```python
from build123d import *

# Parameters (mm, degrees)
SKETCH1_R           = 114.3
SKETCH1_R_2         = 22.5
SKETCH1_R_3         = 30
BOSS_EXTRUDE1_DEPTH = 50
CUT_EXTRUDE1_START  = -35
SKETCH2_R           = 90
SKETCH2_R_2         = 60
CUT_EXTRUDE1_DEPTH  = 20


with BuildPart() as part:
    # Sketch1 → Boss-Extrude1 (new body)
    with BuildSketch(Plane(origin=(0, 0, 0), x_dir=(1, 0, 0), z_dir=(0, 1, 0))):
        with Locations(Location((0, 0, 0), (0, 0, 270))):
            Circle(SKETCH1_R)
        with Locations(Location((75, 0, 0), (0, 0, 270))):
            Circle(SKETCH1_R_2, mode=Mode.SUBTRACT)
        with Locations(Location((53.031031744, 53.03498536, 0), (0, 0, 270))):
            Circle(SKETCH1_R_2, mode=Mode.SUBTRACT)
        with Locations(Location((0, 75, 0), (0, 0, 270))):
            Circle(SKETCH1_R_2, mode=Mode.SUBTRACT)
        with Locations(Location((-52.573136336, 53.488927226, 0), (0, 0, 270))):
            Circle(SKETCH1_R_2, mode=Mode.SUBTRACT)
        with Locations(Location((-75, 0, 0), (0, 0, 270))):
            Circle(SKETCH1_R_2, mode=Mode.SUBTRACT)
        with Locations(Location((-53.03498536, -53.031031744, 0), (0, 0, 270))):
            Circle(SKETCH1_R_2, mode=Mode.SUBTRACT)
        with Locations(Location((0, -75, 0), (0, 0, 270))):
            Circle(SKETCH1_R_2, mode=Mode.SUBTRACT)
        with Locations(Location((53.488927226, -52.573136336, 0), (0, 0, 270))):
            Circle(SKETCH1_R_2, mode=Mode.SUBTRACT)
        with Locations(Location((0, 0, 0), (0, 0, 270))):
            Circle(SKETCH1_R_3, mode=Mode.SUBTRACT)
    extrude(amount=BOSS_EXTRUDE1_DEPTH)

    # Sketch2 → Cut-Extrude1 (cut)
    with BuildSketch(Plane(origin=(0, 50, 0), x_dir=(1, 0, 0), z_dir=(0, 1, 0)).offset(CUT_EXTRUDE1_START)):
        Circle(SKETCH2_R)
        Circle(SKETCH2_R_2, mode=Mode.SUBTRACT)
    extrude(amount=-CUT_EXTRUDE1_DEPTH, mode=Mode.SUBTRACT)


solid = part.part
```
The listing builds one solid part. Answer for the finished solid, in the listing's coordinates (mm). A direction names the side the tool comes from. Coordinates: 2 decimals unless noted, no trailing zeros. Loops run counter-clockwise (first coordinate to the right, second up) from the corner with the lowest first, then second, coordinate; pieces in that order, holes last. Notation, with made-up numbers: M 89.5,0.5 L 96.5,0.5 A23 cw 96.5,29.5 Z; hole C -39,27.25 d4. An arc over 180 degrees is marked long. Answer as CSV lines item,"result". Start each with the question number.
(1) The part is cut by section A-A (x = 0). Give the vertices of the cut face in (y, z).
(2) The part is cut by section D-D (z = -92). Give the vertices of the cut face in (x, y), and give its area (3 significant figures).
(3) The part is cut by section B-B (y = 5.5). State how many separate pieces and enclosed holes the cut face has, and give its area (3 significant figures).
(4) The mould has two halves that part along Z. Classify faces 3 (the flat face through (70, 15, -29)), 4 (the cylindrical face through (5.03, 24.65, -114.19)), 5 (the flat face through (27, 0, -27)): pulls with the +Z half, pulls with the -Z half, needs draft (parallel to the pull), parting line crosses it, or undercut.
(5) Given pin 1 (10 mm diameter, centred on x = 7, y = 41.5, fed in from -Z); pin 2 (1.5 mm diameter, centred on y = 43.5, z = -78.5, fed in from -X); pin 3 (1 mm diameter, centred on x = 70, y = 23, fed in from -Z), each flat-ended and moving along its own axis, determine where each tip first touches the part or whether it passes through.
(6) Find the intervals of material crossed by L1, parallel to X at y = 24, z = 0; L2, parallel to Z at x = -67, y = 46; L3, parallel to Z at x = -50.5, y = 30, in increasing order. Write a range as [from, to].
(7) The part is cut by section C-C (z = 0). Give the vertices of the cut face in (x, y), and give its area (3 significant figures).
(8) For faces 1 (the flat face through (28, 15, -70)), 2 (the cylindrical face through (72.46, 30.21, 64.67)), determine the directions among +Z, -Z, +X, -X, +Y, -Y from which every point of the face is accessible in a straight line to the end or side of a thin tool.
Determined:
1,outline,"M 0,-114.3 L 50,-114.3 L 50,-97.5 L 0,-97.5 Z; M 0,-52.5 L 50,-52.5 L 50,-30 L 0,-30 Z; M 0,30 L 50,30 L 50,52.5 L 0,52.5 Z; M 0,97.5 L 50,97.5 L 50,114.3 L 0,114.3 Z"
2,outline,"M -67.83,0 L -14.74,0 L -14.74,50 L -67.83,50 Z; M 14.74,0 L 67.83,0 L 67.83,50 L 14.74,50 Z"
2,area,"5,310 mm2"
3,separate pieces,"2"
3,enclosed holes,"2"
3,area,"21,300 mm2"
4,face 3,"undercut"
4,face 4,"parting line crosses it"
4,face 5,"needs draft"
5,pin 1,"z = -114.28"
5,pin 2,"x = -83.78"
5,pin 3,"z = -90.74"
6,L1,"[-114.3, -97.5], [-52.5, -30], [30, 52.5], [97.5, 114.3]"
6,L2,"[-92.6, -70.75], [-36.22, -21.03], [21.03, 35.39], [70.67, 92.6]"
6,L3,"[-102.54, -75.89], [-31.08, 30.67], [75.39, 102.54]"
7,outline,"M -114.3,0 L -97.5,0 L -97.5,50 L -114.3,50 Z; M -52.5,0 L -30,0 L -30,50 L -52.5,50 Z; M 30,0 L 52.5,0 L 52.5,50 L 30,50 Z; M 97.5,0 L 114.3,0 L 114.3,50 L 97.5,50 Z"
7,area,"3,930 mm2"
8,face 1,"-Y"
8,face 2,"+Y, -Y"
